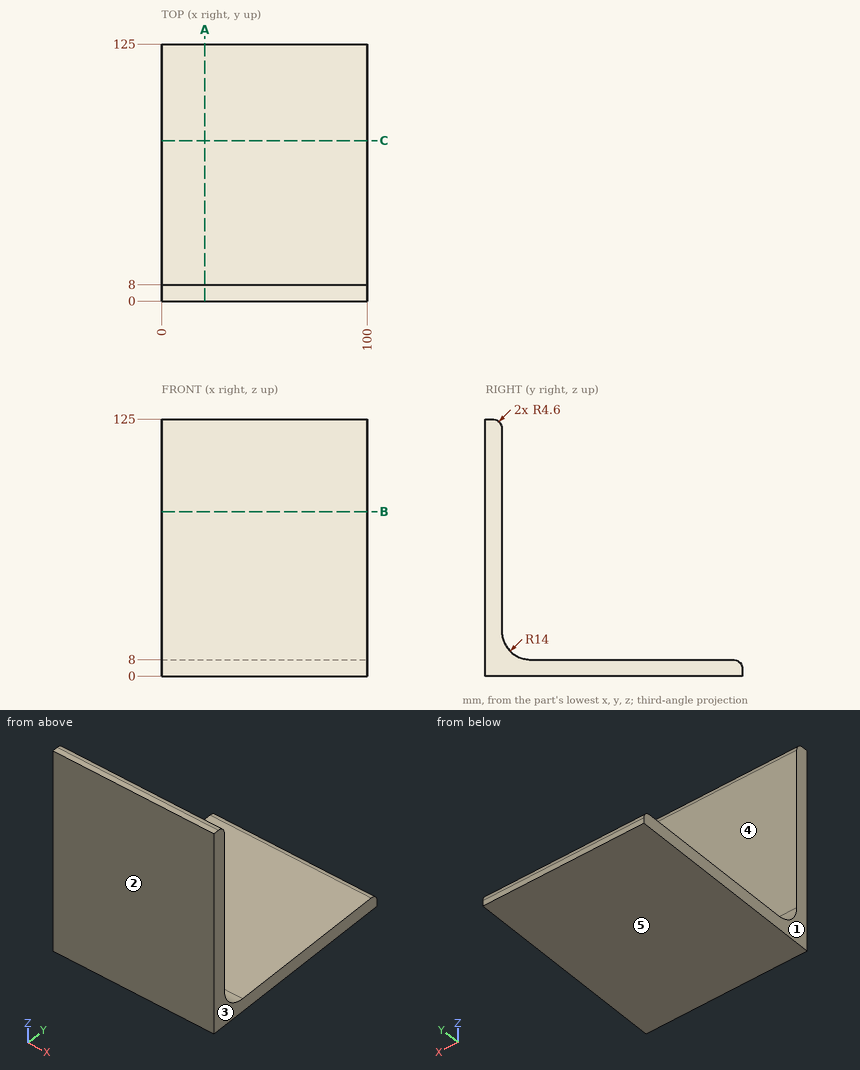
Could you check a few things on this drawing? It's one solid part, dimensions in mm from its lowest x, y, z. A direction names the side the tool comes from. Coordinates: 2 decimals unless noted, no trailing zeros. Order: outer loops, then holes, each group sorted by start corner. A loop starts at its lowest first (then second) coordinate and runs counter-clockwise, first axis right, second up. Notation, with made-up numbers: M 86,35 L 130,35 A11 cw 130,50 Z; hole C 23.25,34 d7. An arc over 180 degrees is marked long. Answer as a JSON object with one key per item and string values. Group by question number.
(1) Suppose I cut it at B-B, the plane z = 80. Please give me the cut outline in (x, y).
(2) If we mould it in two halves opening along X, with no side actions, what happens to the marked faces 1, 2 and 3? For each: released by +X, released by -X, zero draft, split by the parting line, or undercut.
(3) I need wall thicknesses on probe 1 along Z at (x, y) = (76, 89.5); probe 2 along Z at (x, y) = (43, 10.5). Which ranges of each line are inside material? Lowest first, please.
(4) Which directions (+Z, -Z, +X, -X, +Y, -Y) give clear straight access to the entire face, cutting with the end or side of a thin tool? Please do the marked faces 4 and 5.
(5) Suppose I cut it at A-A, the plane x = 21. Please give me the cut outline in (y, z), then the cut area to 3 significant figures.
(6) For pin 1 (1.5 mm diameter, centred on x = 37.5, z = 47.5, fed in from +Y), with a flat end and sliding along its axis, tell me the tip position at first contact or that it passes through.
Values found:
{
 "1": {"outline": "M 0,0 L 100,0 L 100,8 L 0,8 Z"},
 "2": {"face 1": "released by -X", "face 2": "zero draft", "face 3": "released by +X"},
 "3": {"probe 1": "z = 0 to 8", "probe 2": "z = 0 to 14.02"},
 "4": {"face 4": "+Z, +X, -X, +Y", "face 5": "-Z, +X, -X, +Y, -Y"},
 "5": {"outline": "M 0,0 L 125,0 L 125,3.4 A4.6 ccw 120.4,8 L 22,8 A14 cw 8,22 L 8,120.4 A4.6 ccw 3.4,125 L 0,125 Z", "area": "1,970 mm^2"},
 "6": {"pin 1": "stops at y = 8"}
}
